Geometry check sheet. Reference: the model listing, model coordinates, mm. Face numbers are marked on the shaded views. A direction names the side the tool comes from. Round coordinates to 2 decimals unless told otherwise and drop trailing zeros. Order: outer loops, then holes, each group sorted by start corner. A loop starts at its lowest first (then second) coordinate and runs counter-clockwise, first axis right, second up. Notation, with made-up numbers: (61.5, 22) - (67.5, 22) arc R25 ccw to (67.5, 52) - close; hole circle Ø1 at (57.25, 62). An arc over 180 degrees is marked (long way). Write each question's results on one line, items separated by ' | '.
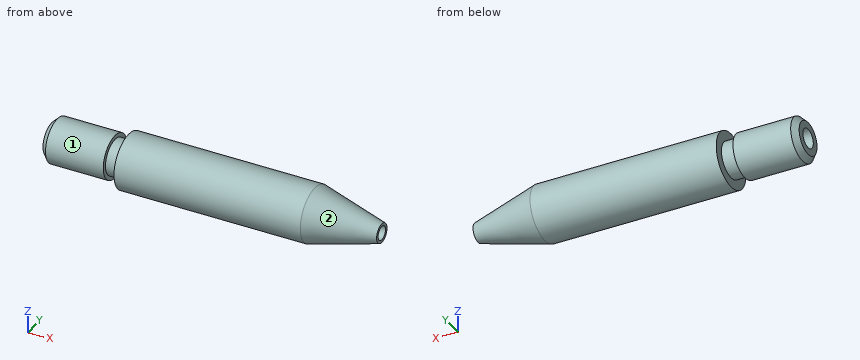
```python
from build123d import *

# Parameters (mm, degrees)
SKETCH_2_R          = 1.75
CUT_EXTRUDE_2_DEPTH = 56
SKETCH_3_R          = 1.25
CUT_EXTRUDE_3_DEPTH = 61.415229868
CHAMFER_1_SIZE      = 1


with BuildPart() as part:
    # 草图1 → 旋转2 (revolve)
    with BuildSketch(Plane.XY, mode=Mode.PRIVATE) as revolve_2_sk:
        Polygon((-8.728334407, 0), (-49.046975166, 0), (-49.046975166, 4), (-37.546975166, 4), (-37.546975166, 3.25), (-35.046975166, 3.25), (-35.046975166, 5), (-1.17614029, 5), (10.953024834, 1.75), (10.953024834, 0), align=None)
    revolve(revolve_2_sk.sketch.rotate(Axis((-15.390186902, 0, 0), (1, 0, 0)), 90), axis=Axis((-15.390186902, 0, 0), (1, 0, 0)))

    # 草图2 → 切除-拉伸2 (cut)
    with BuildSketch(Plane.ZY.offset(49.046975166)):
        Circle(SKETCH_2_R)
    extrude(amount=-CUT_EXTRUDE_2_DEPTH, mode=Mode.SUBTRACT)

    # 草图3 → 切除-拉伸3 (cut, through all)
    with BuildSketch(Plane(origin=(10.953024834, 0, 0), x_dir=(0, 0, -1), z_dir=(1, 0, 0))):
        Circle(SKETCH_3_R)
    extrude(amount=-CUT_EXTRUDE_3_DEPTH, mode=Mode.SUBTRACT)

    # 倒角1
    chamfer_1_edges = [part.edges().sort_by_distance(p)[0] for p in [
        (-49.046975166, 0, -4),
    ]]
    chamfer(chamfer_1_edges, length=CHAMFER_1_SIZE)


solid = part.part
```
(1) Section check D-D (x = -38.5). Record the cut outline in (y, z), then the cut area to 3 significant figures.
Answers follow:
outline: circle Ø8 at (0, 0); hole circle Ø3.5 at (0, 0) | area: 40.6 mm²
(2) Section check C-C (x = -20.5). Record the cut outline in (y, z).
Answers follow:
outline: circle Ø10 at (0, 0); hole circle Ø3.5 at (0, 0)
(3) Depth check by flat-ended pin: pin 1 Ø6 at (x, y) = (0, -3) entering from +Z; pin 2 Ø3 at (y, z) = (0, 0) entering from -X; pin 3 Ø1.5 at (x, y) = (-40, -2) entering from +Z. Enter the tip coordinate at first touch or a pass-through.
Answers follow:
pin 1: z = 4.99 | pin 2: x = 6.95 | pin 3: z = 3.8
(4) Material ranges on line 1 (Y direction, x = -34, z = 0); line 2 (Y direction, x = -37, z = 0); line 3 (Z direction, x = -12.5, y = -0.5), recorded low to high.
Answers follow:
line 1: -5 to -1.75, 1.75 to 5 | line 2: -3.25 to -1.75, 1.75 to 3.25 | line 3: -4.97 to -1.68, 1.68 to 4.97
(5) Section check A-A (z = 0). Record the cut outline in (x, y).
Answers follow:
outline: (-49.05, -3) - (-48.05, -4) - (-37.55, -4) - (-37.55, -3.25) - (-35.05, -3.25) - (-35.05, -5) - (-1.18, -5) - (10.95, -1.75) - (10.95, -1.25) - (6.95, -1.25) - (6.95, -1.75) - (-49.05, -1.75) - close; (-49.05, 1.75) - (6.95, 1.75) - (6.95, 1.25) - (10.95, 1.25) - (10.95, 1.75) - (-1.18, 5) - (-35.05, 5) - (-35.05, 3.25) - (-37.55, 3.25) - (-37.55, 4) - (-48.05, 4) - (-49.05, 3) - close
(6) Access from +Z, -Z, +X, -X, +Y, -Y to the whole of each face (thin tool, end or side, straight path). Record for the marked faces 1 and 2.
Answers follow:
face 1: -X | face 2: +X
